Geometry check sheet. Reference: the model listing, model coordinates, mm. Coordinates: 2 decimals unless noted, no trailing zeros. Loops run counter-clockwise (first coordinate to the right, second up) from the corner with the lowest first, then second, coordinate; pieces in that order, holes last.
from build123d import *

# Parameters (mm, degrees)
F0_R     = 3.25
F0_R_2   = 3
F0_R_3   = 2.5
F1_DEPTH = 5
F2_SIZE  = 3
F3_SIZE  = 3
F4_SIZE  = 2.5
F5_SIZE  = 2.5


with BuildPart() as f1:
    # F0 (on Top) → F1 (new body)
    with BuildSketch(Plane.XY):
        with BuildLine():
            Line((-42, 0), (0, 0))
            Line((0, 0), (0, 41.5))
            Line((0, 41.5), (-27, 41.5))
            ThreePointArc((-27, 41.5), (-31.393398, 30.893398), (-42, 26.5))
            Line((-42, 26.5), (-42, 0))
        make_face()
        with Locations((-17.2, 18.18)):
            Circle(F0_R, mode=Mode.SUBTRACT)
        with Locations((-25.75, 25.25)):
            Circle(F0_R_2, mode=Mode.SUBTRACT)
        with BuildLine():
            Line((-84, 0), (-42, 0))
            Line((-42, 0), (-42, 26.5))
            ThreePointArc((-42, 26.5), (-52.606602, 30.893398), (-57, 41.5))
            Line((-57, 41.5), (-84, 41.5))
            Line((-84, 41.5), (-84, 0))
        make_face()
        with Locations((-66.8, 18.18)):
            Circle(F0_R, mode=Mode.SUBTRACT)
        with Locations((-58.25, 25.25)):
            Circle(F0_R_2, mode=Mode.SUBTRACT)
        with BuildLine():
            Line((-27, 41.5), (0, 41.5))
            Line((0, 41.5), (0, 83))
            Line((0, 83), (-42, 83))
            Line((-42, 83), (-42, 56.5))
            ThreePointArc((-42, 56.5), (-31.393398, 52.106602), (-27, 41.5))
        make_face()
        with Locations((-25.75, 57.75)):
            Circle(F0_R_2, mode=Mode.SUBTRACT)
        with Locations((-6.5, 70.5)):
            Circle(F0_R_3, mode=Mode.SUBTRACT)
        with BuildLine():
            Line((-84, 83), (-84, 41.5))
            Line((-84, 41.5), (-57, 41.5))
            ThreePointArc((-57, 41.5), (-52.606602, 52.106602), (-42, 56.5))
            Line((-42, 56.5), (-42, 83))
            Line((-42, 83), (-84, 83))
        make_face()
        with Locations((-58.25, 57.75)):
            Circle(F0_R_2, mode=Mode.SUBTRACT)
        with Locations((-77.5, 70.5)):
            Circle(F0_R_3, mode=Mode.SUBTRACT)
    extrude(amount=F1_DEPTH)

    # F2
    f2_edges = [f1.edges().sort_by_distance(p)[0] for p in [
        (-80, 70.5, 5),
    ]]
    chamfer(f2_edges, length=F2_SIZE)

    # F3
    f3_edges = [f1.edges().sort_by_distance(p)[0] for p in [
        (-9, 70.5, 5),
    ]]
    chamfer(f3_edges, length=F3_SIZE)

    # F4
    f4_edges = [f1.edges().sort_by_distance(p)[0] for p in [
        (-70.05, 18.18, 5),
    ]]
    chamfer(f4_edges, length=F4_SIZE)

    # F5
    f5_edges = [f1.edges().sort_by_distance(p)[0] for p in [
        (-20.45, 18.18, 5),
    ]]
    chamfer(f5_edges, length=F5_SIZE)


solid = f1.part
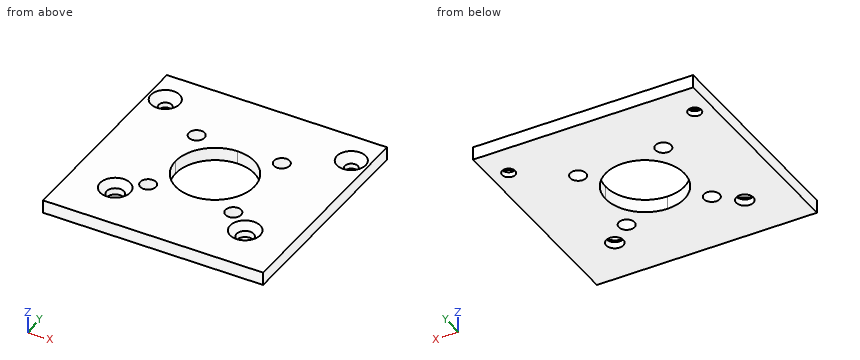
(1) Scan lines: L1, parallel to Y at x = -58.25, z = 1.65; L2, parallel to Y at x = -6.5, z = 0.65; L3, parallel to X at y = 16, z = 4.15. Record each from-to range of solid material in increasing order.
Findings:
L1: y = 0 to 22.25, 28.25 to 54.75, 60.75 to 83
L2: y = 0 to 68, 73 to 83
L3: x = -84 to -71.19, -62.41 to -21.59, -12.81 to 0
(2) Sectioned sample at B-B on y = 57.75. Record the cut outline in (x, z), and give its area (3 significant figures).
Findings:
outline: (-84, 0) - (-61.25, 0) - (-61.25, 5) - (-84, 5) - close; (-55.25, 0) - (-28.75, 0) - (-28.75, 5) - (-55.25, 5) - close; (-22.75, 0) - (0, 0) - (0, 5) - (-22.75, 5) - close
area: 360 mm2
(3) Sectioned sample at D-D on y = 18.18. Record the cut outline in (x, z).
Findings:
outline: (-84, 0) - (-70.05, 0) - (-70.05, 2.5) - (-72.55, 5) - (-84, 5) - close; (-63.55, 0) - (-20.45, 0) - (-20.45, 2.5) - (-22.95, 5) - (-61.05, 5) - (-63.55, 2.5) - close; (-13.95, 0) - (0, 0) - (0, 5) - (-11.45, 5) - (-13.95, 2.5) - close
(4) Gauge pin test, flat ends, axial feed: pin 1 Ø6 at (x, y) = (-6.5, 70.5) entering from +Z; pin 2 Ø4 at (x, y) = (-17.2, 18.18) entering from +Z. Record the tip position at first contact, or that the pin passes through.
Findings:
pin 1: stops at z = 2.5
pin 2: passes through
(5) Sectioned sample at A-A on z = 0.75. State how many separate pieces and enclosed holes the cut face has, and give its area (3 significant figures).
Findings:
separate pieces: 1
enclosed holes: 9
area: 6,050 mm2
(6) Sectioned sample at C-C on x = -66.8. Record the cut outline in (y, z).
Findings:
outline: (0, 0) - (14.93, 0) - (14.93, 2.5) - (12.43, 5) - (0, 5) - close; (21.43, 0) - (83, 0) - (83, 5) - (23.93, 5) - (21.43, 2.5) - close
